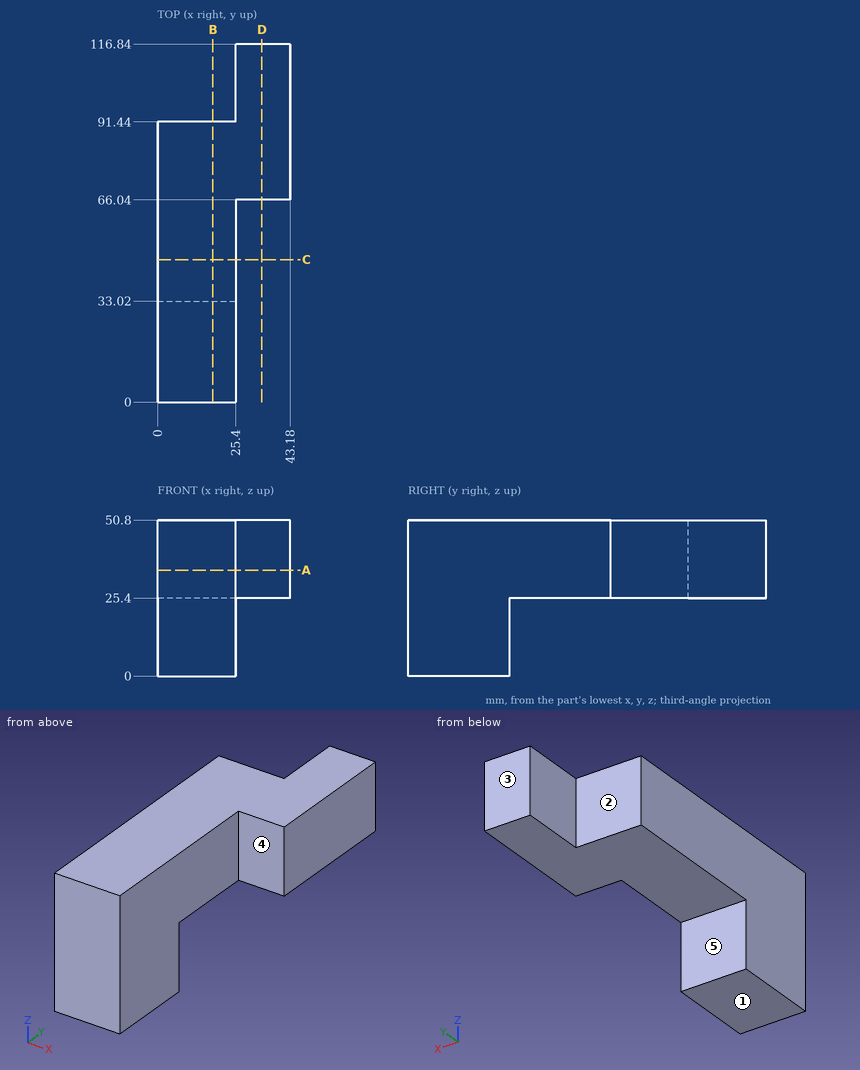
Here's the drawing with two shaded views (mm, measured from the low corner). I have some questions. A direction names the side the tool comes from. Give positions to 0.01 mm unless a question says otherwise; leave off trailing zeros. Write each loop counter-clockwise with the first axis right and the second up, starting at its lowest first coordinate (ties: lowest second). Pieces come first, ordered by that corner, then holes. Notation, with made-up numbers: (-27.75, -5.75) -> (10.25, -5.75) arc R27 ccw to (10.25, 11.25) -> close; hole circle Ø8 at (-7, 52). An arc over 180 degrees is marked (long way). Use one line per item in the form item = value.
1) Suppose I cut it at B-B (x = 18). Please give me the cut outline in (y, z).
Verdict:
outline = (0, 0) -> (33.02, 0) -> (33.02, 25.4) -> (91.44, 25.4) -> (91.44, 50.8) -> (0, 50.8) -> close
2) Suppose I cut it at C-C (y = 46.5). Please give me the cut outline in (x, z).
Verdict:
outline = (0, 25.4) -> (25.4, 25.4) -> (25.4, 50.8) -> (0, 50.8) -> close
3) I'm going to push flat-ended pins straight in: pin 1 (9 mm diameter, centred on x = 36.5, z = 41, fed in from -Y); pin 2 (5 mm diameter, centred on x = 11, z = 18.5, fed in from +Y); pin 3 (7.5 mm diameter, centred on y = 109.5, z = 43, fed in from -X). Where does each tip first touch, or does it pass through?
Verdict:
pin_1 = 66.04
pin_2 = 33.02
pin_3 = 25.4
4) On a 3-axis mill with a long thin cutter (end or side, diameter ignored), from which of +Z, -Z, +X, -X, +Y, -Y can I reach the whole of each face in a straight line? I mean the marked faces 1, 2, 3, 4 and 5. Say none if no direction works.
Verdict:
face_1 = -Z, +X, -X, +Y, -Y
face_2 = +Z, -Z, -X, +Y
face_3 = +Z, -Z, +X, -X, +Y
face_4 = +Z, -Z, +X, -Y
face_5 = -Z, +X, -X, +Y
5) Suppose I cut it at D-D (x = 34). Please give me the cut outline in (y, z).
Verdict:
outline = (66.04, 25.4) -> (116.84, 25.4) -> (116.84, 50.8) -> (66.04, 50.8) -> close
6) If I drill on L1, parallel to Y at x = 11, z = 46; L2, parallel to Z at x = 3, y = 50.5; L3, parallel to Y at x = 28.5, z = 42, over which ranges is the centre line in solid material (lowest first)? Write a range as [from, to].
Verdict:
L1 = [0, 91.44]
L2 = [25.4, 50.8]
L3 = [66.04, 116.84]
7) Suppose I cut it at A-A (z = 34.5). Please give me the cut outline in (x, y).
Verdict:
outline = (0, 0) -> (25.4, 0) -> (25.4, 66.04) -> (43.18, 66.04) -> (43.18, 116.84) -> (25.4, 116.84) -> (25.4, 91.44) -> (0, 91.44) -> close
